Part model, mm, in its own coordinate system. Face numbers are marked on the shaded views. A direction names the side the tool comes from. Round coordinates to 2 decimals unless told otherwise and drop trailing zeros. Order: outer loops, then holes, each group sorted by start corner. A loop starts at its lowest first (then second) coordinate and runs counter-clockwise, first axis right, second up. Notation, with made-up numbers: (-22, 55) -> (-18, 55) arc R21 cw to (-18, 91) -> close; hole circle Ø11 at (-38.5, 76). An arc over 180 degrees is marked (long way). Return JSON: item names as keys, results as strings. Group by question number.
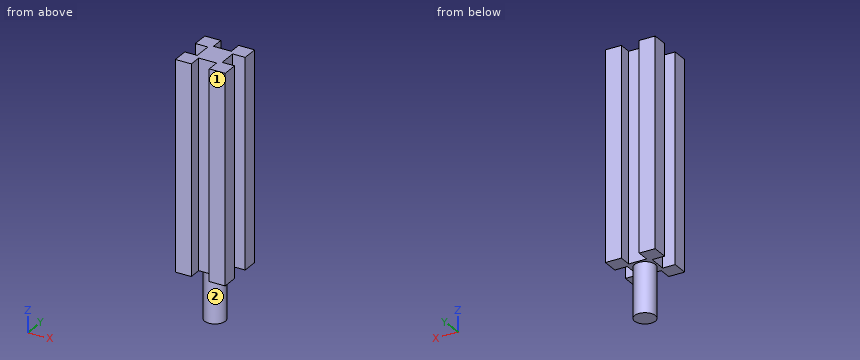
Autodesk Fusion 360 part; units mm, degrees
sketch "Sketch1" plane through (0, 0, 0) normal (0, 0, 1) x (1, 0, 0) in component "Pillar"
  line L0 (6, -6) -> (-6, -6)
  line L1 (-6, -6) -> (-6, 6)
  line L2 (-6, 6) -> (6, 6)
  line L3 (6, 6) -> (6, -6)
  line L4 (6, -6) -> (-6, 6) construction
  line L5 (-6, -6) -> (6, 6) construction
  dimension "d1" = 12
  dimension "d2" = 12
extrude "Extrude1" add sketch "Sketch1" along normal blind 50 in component "Pillar"
sketch "Sketch2" plane through (0, 0, 50) normal (0, 0, 1) x (-1, 0, 0) in component "Pillar"
  line L0 (-6, -6) -> (6, -6)
  line L1 (6, -6) -> (6, 6)
  line L2 (6, 6) -> (-6, 6)
  line L3 (-6, 6) -> (-6, -6)
  line L4 (-3, 2.15) -> (-9, 2.15)
  line L5 (-9, 2.15) -> (-9, -2.15)
  line L6 (-9, -2.15) -> (-3, -2.15)
  line L7 (-3, -2.15) -> (-3, 2.15)
  line L8 (-3, 2.15) -> (-9, -2.15) construction
  line L9 (-9, 2.15) -> (-3, -2.15) construction
  line L10 (2.15, -9) -> (-2.15, -9)
  line L11 (-2.15, -9) -> (-2.15, -3)
  line L12 (-2.15, -3) -> (2.15, -3)
  line L13 (2.15, -3) -> (2.15, -9)
  line L14 (2.15, -9) -> (-2.15, -3) construction
  line L15 (-2.15, -9) -> (2.15, -3) construction
  line L16 (9, -2.15) -> (3, -2.15)
  line L17 (3, -2.15) -> (3, 2.15)
  line L18 (3, 2.15) -> (9, 2.15)
  line L19 (9, 2.15) -> (9, -2.15)
  line L20 (9, -2.15) -> (3, 2.15) construction
  line L21 (3, -2.15) -> (9, 2.15) construction
  line L22 (-2.15, 9) -> (2.15, 9)
  line L23 (2.15, 9) -> (2.15, 3)
  line L24 (2.15, 3) -> (-2.15, 3)
  line L25 (-2.15, 3) -> (-2.15, 9)
  line L26 (-2.15, 9) -> (2.15, 3) construction
  line L27 (2.15, 9) -> (-2.15, 3) construction
  point P0 (-6, 0)
  point P1 (0, -6)
  point P2 (6, 0)
  point P3 (0, 6)
  dimension "d5" = 6
  dimension "d6" = 4.3
  dimension "d9" = 4.3
  dimension "d10" = 6
  dimension "d11" = 6
  dimension "d12" = 4.3
  dimension "d13" = 4.3
  dimension "d14" = 6
extrude "Extrude7" cut sketch "Sketch2" against normal blind 50 contours L0 L11 L12 L13 | L3 L4 L6 L7 | L1 L16 L17 L18 | L2 L23 L24 L25 in component "Pillar"
extrude "Extrude3" cut sketch "Sketch2" against normal blind 30 contours L0 L11 L12 L13 in component "Pillar"
extrude "Extrude2" cut sketch "Sketch2" against normal blind 30 contours L3 L4 L6 L7 in component "Pillar"
extrude "Extrude4" cut sketch "Sketch2" against normal blind 30 contours L1 L16 L17 L18 in component "Pillar"
extrude "Extrude5" cut sketch "Sketch2" against normal blind 30 contours L2 L23 L24 L25 in component "Pillar"
sketch "Sketch3" plane through (0, 0, 0) normal (0, 0, -1) x (1, 0, 0) in component "Pillar"
  line L0 (2.15, -6) -> (6, -6)
  line L1 (6, -6) -> (6, -2.15)
  line L2 (6, 6) -> (2.15, 6)
  line L3 (-6, 6) -> (-6, 2.15)
  circle A0 centre (0, 0) radius 2.5
  line L4 (-2.15, -6) -> (-2.15, -3)
  line L5 (-2.15, -3) -> (2.15, -3)
  line L6 (2.15, -3) -> (2.15, -6)
  line L7 (6, -2.15) -> (3, -2.15)
  line L8 (3, -2.15) -> (3, 2.15)
  line L9 (3, 2.15) -> (6, 2.15)
  line L10 (6, 2.15) -> (6, 6)
  line L11 (2.15, 6) -> (2.15, 3)
  line L12 (2.15, 3) -> (-2.15, 3)
  line L13 (-2.15, 3) -> (-2.15, 6)
  line L14 (-2.15, 6) -> (-6, 6)
  line L15 (-6, 2.15) -> (-3, 2.15)
  line L16 (-3, 2.15) -> (-3, -2.15)
  line L17 (-3, -2.15) -> (-6, -2.15)
  line L18 (-6, -2.15) -> (-6, -6)
  line L19 (-6, -6) -> (-2.15, -6)
  dimension "d21" = 5
extrude "Extrude6" add sketch "Sketch3" along normal blind 12 contours A0 in component "Pillar"
component "Pillar" placed x (1, 0, 0) y (0, 1, 0) z (0, 0, 1) at (0, 0, 0)
(1) Pin check, flat tips, straight feed: P1, Ø1.3, axis at x = 1, z = 32.5, coming from the +Y side; P2, Ø3, axis at y = 4.5, z = -4, coming from the +X side. Stop position of each tip, or through.
(2) Saw through at C-C, the plane z = 8.5. List the corners of the cut face in (x, y), and give its area (3 significant figures).
(3) Saw through at A-A, the plane y = 5. List the corners of the cut face in (x, z), and give its area (3 significant figures).
(4) Tool access for the marked faces 1 and 2: list every direction of +Z, -Z, +X, -X, +Y, -Y with a clear straight run to the whole face (end or side of a thin tool).
(5) Probe L1, parallel to Y at x = -3.5, z = 2; L2, parallel to Y at x = -0.5, z = 20.5. List the from-to ranges inside material, lowest first. Write a range as [from, to].
(6) Saw through at B-B, the plane x = 0. List the corners of the cut face in (y, z), and give its area (3 significant figures).
Results are:
{
 "1": {"P1": "stops at y = 3", "P2": "passes through"},
 "2": {"outline": "(-6, -6) -> (-2.15, -6) -> (-2.15, -3) -> (2.15, -3) -> (2.15, -6) -> (6, -6) -> (6, -2.15) -> (3, -2.15) -> (3, 2.15) -> (6, 2.15) -> (6, 6) -> (2.15, 6) -> (2.15, 3) -> (-2.15, 3) -> (-2.15, 6) -> (-6, 6) -> (-6, 2.15) -> (-3, 2.15) -> (-3, -2.15) -> (-6, -2.15) -> close", "area": "92.4 mm^2"},
 "3": {"outline": "(-6, 0) -> (-2.15, 0) -> (-2.15, 50) -> (-6, 50) -> close; (2.15, 0) -> (6, 0) -> (6, 50) -> (2.15, 50) -> close", "area": "385 mm^2"},
 "4": {"face 1": "+Z, -Z, +X, -X, -Y", "face 2": "-Z"},
 "5": {"L1": "y = [-6, -2.15], [2.15, 6]", "L2": "y = [-3, 3]"},
 "6": {"outline": "(-3, 0) -> (-2.5, 0) -> (-2.5, -12) -> (2.5, -12) -> (2.5, 0) -> (3, 0) -> (3, 50) -> (-3, 50) -> close", "area": "360 mm^2"}
}
